Verification items for the finished model (mm, model axes). A direction names the side the tool comes from. Give positions to 0.01 mm unless a question says otherwise; leave off trailing zeros. Order: outer loops, then holes, each group sorted by start corner. A loop starts at its lowest first (then second) coordinate and runs counter-clockwise, first axis right, second up. Notation, with made-up numbers: (27, -27) - (69, -27) arc R22 cw to (69, 6) - close; hole circle Ø7 at (-30.75, 69.25). An arc over 180 degrees is marked (long way). Answer as a JSON object with one key per item and string values. Group by question number.
(1) Mould release check, pull along Y, two halves, no side actions. Record for faces 1 (the face through (13, 1.75, 4)), 2 (the face through (6, 3, 8.25)), 3 (the face through (20.46, 4.03, 1.88)), 4 (the face through (21, 8, 5)): +Y half, -Y half, draft (parallel to the pull), parting line (faces both ways), or undercut.
(2) Section check A-A (y = 1.5). Record the boundary of the cut face in (x, z), then the cut area to 4 significant figures.
(3) Section check B-B (z = 3.25). Count the separate pieces of the cut face and the enclosed holes in it, then the cut area to 3 significant figures.
(4) Access from +Z, -Z, +X, -X, +Y, -Y to the whole of each face (thin tool, end or side, straight path). Record for faces 5 (the face through (23.8, 8.2, 5.5)), 6 (the face through (2.8, 8.2, 5.5)), 7 (the face through (7.42, 2.42, 6.35)), 8 (the face through (13.573, 7.398, 2.184)), 9 (the face through (2, 4, 5)).
(5) Thickness scan on line 1 (Y direction, x = 10, z = 5); line 2 (Z direction, x = 3.5, y = 3.5); line 3 (Z direction, x = 13.5, y = 6). Record the ranges inside material, lowest first.
(6) Depth check by flat-ended pin: pin 1 Ø0.9 at (x, y) = (20.59, 4) entering from +Z; pin 2 Ø0.8 at (x, z) = (8, 5) entering from -Y; pin 3 Ø0.6 at (x, y) = (25, 5) entering from +Z. Enter the tip coordinate at first touch or a pass-through.
Autodesk Inventor part; units mm, degrees
ref_plane "YZ Plane" through (0, 0, 0) normal (1, 0, 0) x (0, 1, 0)
ref_plane "XZ Plane" through (0, 0, 0) normal (0, 1, 0) x (-1, 0, 0)
ref_plane "XY Plane" through (0, 0, 0) normal (0, 0, 1) x (1, 0, 0)
sketch "Sketch1" plane through (0, 0, 0) normal (0, 0, 1) x (1, 0, 0)
  line L0 (0, 0) -> (27, 0)
  line L1 (27, 0) -> (27, 9)
  line L2 (27, 9) -> (0, 9)
  line L3 (0, 9) -> (0, 0)
  dimension "d0" = 27
  dimension "d1" = 9
extrude "Extrusion1" add sketch "Sketch1" along normal blind 5
sketch "Sketch2" plane through (0, 0, 5) normal (0, 0, 1) x (1, 0, 0)
  line L0 (0, 0) -> (27, 0)
  line L1 (0, 0) -> (1, 0)
  line L2 (1, 0) -> (1, 8)
  line L3 (1, 8) -> (26, 8)
  line L4 (26, 8) -> (26, 0)
  line L5 (27, 0) -> (27, 9)
  line L6 (27, 0) -> (26, 0)
  line L7 (27, 0) -> (27, 9)
  line L8 (27, 9) -> (0, 9)
  line L9 (0, 9) -> (0, 0)
  line L10 (0, 9) -> (0, 0)
  line L11 (13.5, 12) -> (13.5, -6.262) construction
  dimension "d4" = 1
  dimension "d5" = 1
extrude "Extrusion2" add sketch "Sketch2" along normal blind 0.5 contours L9 L8 L5 L0 L4 L3 L2
sketch "Sketch3" plane through (0, 0, 5) normal (0, 0, 1) x (1, 0, 0)
  line L0 (26, 0) -> (26, 8) construction
  line L1 (26, 8) -> (1, 8) construction
  line L2 (1, 8) -> (1, 0) construction
  line L3 (1, 0) -> (26, 0) construction
  line L4 (0, 0) -> (1, 0) construction
  line L5 (1, 0) -> (1, 8) construction
  line L6 (1, 8) -> (26, 8) construction
  line L7 (26, 8) -> (26, 0) construction
  line L8 (26, 0) -> (27, 0) construction
  line L9 (27, 0) -> (27, 9) construction
  line L10 (27, 9) -> (0, 9) construction
  line L11 (0, 9) -> (0, 0) construction
  line L12 (3, 0) -> (24, 0)
  line L13 (0, 0) -> (27, 0)
  line L14 (3, 0) -> (3, 8)
  line L15 (24, 0) -> (24, 8)
  line L16 (13.5, 10.7744) -> (13.5, -2.6721) construction
  line L17 (3, 8) -> (24, 8)
  dimension "d8" = 21
extrude "Extrusion3" cut sketch "Sketch3" against normal blind 0.5
sketch "Sketch4" plane through (0, 0, 4.5) normal (0, 0, 1) x (1, 0, 0)
  line L0 (24, 0) -> (3, 0) construction
  line L1 (24, 8) -> (24, 0) construction
  line L2 (3, 8) -> (24, 8) construction
  line L3 (3, 0) -> (3, 8) construction
  line L4 (3, 0) -> (3, 8) construction
  line L5 (3, 8) -> (1, 8) construction
  line L6 (1, 8) -> (1, 0) construction
  line L7 (1, 0) -> (3, 0) construction
  line L8 (24, 8) -> (24, 0) construction
  line L9 (24, 0) -> (26, 0) construction
  line L10 (26, 0) -> (26, 8) construction
  line L11 (26, 8) -> (24, 8) construction
  line L12 (0, 0) -> (1, 0) construction
  line L13 (1, 0) -> (1, 8) construction
  line L14 (1, 8) -> (26, 8) construction
  line L15 (26, 8) -> (26, 0) construction
  line L16 (26, 0) -> (27, 0) construction
  line L17 (27, 0) -> (27, 9) construction
  line L18 (27, 9) -> (0, 9) construction
  line L19 (0, 9) -> (0, 0) construction
  line L20 (13.5, 12.5235) -> (13.5, -4.7396) construction
  circle A0 centre (6.4125, 4) radius 1.875
  circle A1 centre (20.5875, 4) radius 1.875
  point P0 (13.5, 10.4822)
  dimension "d12" = 4
  dimension "d13" = 14.175
  dimension "d14" = 3.75
extrude "Extrusion4" add sketch "Sketch4" along normal blind 3.75
sketch "Sketch5" plane through (6.4125, 4, 8.25) normal (0, 0, 1) x (1, 0, 0)
  circle A0 centre (0, 0) radius 1.875
  circle A1 centre (14.175, 0) radius 1.875
  point P0 (-6.4125, -4)
hole "Hole1" at (6.4125, 4, 8.25) at (20.5875, 4, 8.25) direction (0, 0, -1) diameter 1.5 depth 6 tip angle 118
sketch "Sketch7" plane through (0, 0, 5.5) normal (0, 0, 1) x (1, 0, 0)
  line L0 (0, 0) -> (1, 0) construction
  line L1 (1, 0) -> (1, 8) construction
  line L2 (1, 8) -> (26, 8) construction
  line L3 (26, 8) -> (26, 0) construction
  line L4 (26, 0) -> (27, 0) construction
  line L5 (27, 0) -> (27, 9) construction
  line L6 (27, 9) -> (0, 9) construction
  line L7 (0, 9) -> (0, 0) construction
  circle A0 centre (6.4125, 4) radius 1.875 construction
  circle A1 centre (20.5875, 4) radius 1.875 construction
  line L8 (24, 0) -> (3, 0) construction
  line L9 (24, 8) -> (24, 0) construction
  line L10 (3, 8) -> (24, 8) construction
  line L11 (3, 0) -> (3, 8) construction
  line L12 (24, 8) -> (24, 0) construction
  line L13 (24, 0) -> (26, 0) construction
  line L14 (26, 0) -> (26, 8) construction
  line L15 (26, 8) -> (24, 8) construction
  line L16 (3, 0) -> (3, 8) construction
  line L17 (3, 8) -> (1, 8) construction
  line L18 (1, 8) -> (1, 0) construction
  line L19 (1, 0) -> (3, 0) construction
  line L20 (27, 9) -> (0, 9) construction
  line L21 (13.5, 9) -> (13.5, 1.75)
  line L22 (23, 1.75) -> (16.5, 1.75) construction
  arc A2 (16.5, 1.75) -> (16.8166, 5.75) centre (13.5, 4) ccw
  line L23 (16.5, 1.75) -> (13.5, 1.75)
  line L24 (13.5, 1.75) -> (5.7709, 1.75) construction
  line L25 (16.8166, 5.75) -> (16.8166, 9)
  line L26 (16.8166, 9) -> (13.5, 9)
  line L27 (13.5, 1.75) -> (13.5, 0) construction
  dimension "d28" = 1.75
  dimension "d29" = 3.75
  dimension "d30" = 4
  dimension "d31" = 3
revolve "Revolution1" cut sketch "Sketch7" angle 360 about axis through (13.5, 9, 5.5) along (0, -1, 0)
properties part number "Part2v2"
Solutions:
{
 "1": {"face 1": "+Y half", "face 2": "draft", "face 3": "undercut", "face 4": "undercut"},
 "2": {"outline": "(0, 0) - (27, 0) - (27, 5.5) - (26, 5.5) - (26, 5) - (24, 5) - (24, 4.5) - (3, 4.5) - (3, 5) - (1, 5) - (1, 5.5) - (0, 5.5) - close", "area": "125.5 mm2"},
 "3": {"separate pieces": "1", "enclosed holes": "2", "area": "202 mm2"},
 "4": {"face 5": "+Z, +X, +Y", "face 6": "+Z, -X, +Y", "face 7": "+Z", "face 8": "+Z, +Y", "face 9": "+Z, -Y"},
 "5": {"line 1": "y = 8 to 9", "line 2": "z = 0 to 4.5", "line 3": "z = 0 to 2.18"},
 "6": {"pin 1": "stops at z = 2.07", "pin 2": "stops at y = 2.55", "pin 3": "stops at z = 5"}
}
